For this review, take the finished solid that the model builds, in its own axes (mm). A direction names the side the tool comes from. Round coordinates to 2 decimals unless told otherwise and drop trailing zeros. Order: outer loops, then holes, each group sorted by start corner. A loop starts at its lowest first (then second) coordinate and runs counter-clockwise, first axis right, second up. Notation, with made-up numbers: M 88.5,27 L 141.5,27 A22 ccw 141.5,33 Z; hole C 68,26 d2. An arc over 180 degrees is marked long. Use a Markdown table: item, result.
from build123d import *

# Parameters (mm, degrees)
SKETCH2_W                 = 5
SKETCH2_H                 = 15
BOSS_EXTRUDE1_DEPTH       = 14
BOSS_EXTRUDE1_2_DEPTH     = 14
BOSS_EXTRUDE3_DEPTH       = 25
SKETCH5_W                 = 3
SKETCH5_H                 = 8.8
BOSS_EXTRUDE4_DEPTH       = 14
SKETCH7_W                 = 3
SKETCH7_H                 = 15
BOSS_EXTRUDE5_DEPTH       = 14
SKETCH15_W                = 0.3
SKETCH15_H                = 14
CUT_EXTRUDE2_DEPTH        = 15
SKETCH16_W                = 0.15
SKETCH16_H                = 14
CUT_EXTRUDE3_DEPTH        = 15
FILLET1_R                 = 7
F_4_0MM_DOWEL_HOLE2_D     = 4
FILLET2_R                 = 7
F_4_0MM_DOWEL_HOLE1_D     = 4
F_4_0MM_DOWEL_HOLE1_DEPTH = 26
F_4_0MM_DOWEL_HOLE1_TIP   = 1.201721238
BOSS_EXTRUDE6_DEPTH       = 1
CUT_EXTRUDE4_DEPTH        = 2.4


with BuildPart() as part:
    # Sketch2 → Boss-Extrude1 (new body)
    with BuildSketch(Plane.XY):
        with Locations((-7.5, -1.5)):
            Rectangle(SKETCH2_W, SKETCH2_H)
    extrude(amount=BOSS_EXTRUDE1_DEPTH)



with BuildPart() as body_2:
    # Sketch2 → Boss-Extrude1 2 (new body)
    with BuildSketch(Plane.XY):
        with Locations((7.5, -1.5)):
            Rectangle(SKETCH2_W, SKETCH2_H)
    extrude(amount=BOSS_EXTRUDE1_2_DEPTH)


with BuildPart() as part_1:
    add(part.part)

    add(body_2.part)  # Boss-Extrude3 merges body 2
    # Sketch4 → Boss-Extrude3 (add)
    with BuildSketch(Plane.XY):
        Polygon((-10, 6), (-20, 6), (-22.901603942, 7.206366686), (-26, 7.206366686), (-26, 9.206366686), (-22.502408858, 9.206366686), (-19.600804916, 8), (-10, 8), (10, 8), (19.600804916, 8), (22.502408858, 9.206366686), (26, 9.206366686), (26, 7.206366686), (22.901603942, 7.206366686), (20, 6), (10, 6), align=None)
    extrude(amount=BOSS_EXTRUDE3_DEPTH)

    # Sketch5 → Boss-Extrude4 (add)
    with BuildSketch(Plane.XY):
        with Locations((-11.5, 12.4)):
            Rectangle(SKETCH5_W, SKETCH5_H)
        with Locations((11.5, 12.4)):
            Rectangle(SKETCH5_W, SKETCH5_H)
    extrude(amount=BOSS_EXTRUDE4_DEPTH)

    # Sketch7 → Boss-Extrude5 (add)
    with BuildSketch(Plane.XY):
        with Locations((-14.5, -1.5)):
            Rectangle(SKETCH7_W, SKETCH7_H)
        with Locations((14.5, -1.5)):
            Rectangle(SKETCH7_W, SKETCH7_H)
    extrude(amount=BOSS_EXTRUDE5_DEPTH)

    # Sketch15 → Cut-Extrude2 (cut)
    with BuildSketch(Plane.XZ.offset(9)):
        with Locations((-9.85, 7)):
            Rectangle(SKETCH15_W, SKETCH15_H)
        with Locations((9.85, 7)):
            Rectangle(SKETCH15_W, SKETCH15_H)
        with Locations((-13.15, 7)):
            Rectangle(SKETCH15_W, SKETCH15_H)
        with Locations((13.15, 7)):
            Rectangle(SKETCH15_W, SKETCH15_H)
    extrude(amount=-CUT_EXTRUDE2_DEPTH, mode=Mode.SUBTRACT)

    # Sketch16 → Cut-Extrude3 (cut)
    with BuildSketch(Plane.XZ.offset(9)):
        with Locations((-5.075, 7)):
            Rectangle(SKETCH16_W, SKETCH16_H)
        with Locations((5.075, 7)):
            Rectangle(SKETCH16_W, SKETCH16_H)
    extrude(amount=-CUT_EXTRUDE3_DEPTH, mode=Mode.SUBTRACT)

    # Fillet1
    fillet1_edges = [part_1.edges().sort_by_distance(p)[0] for p in [
        (7.425, -9, 0),
        (7.425, -9, 14),
        (-7.425, -9, 0),
        (-7.425, -9, 14),
        (-14.65, -9, 0),
        (-14.65, -9, 14),
        (14.65, -9, 14),
        (14.65, -9, 0),
    ]]
    fillet(fillet1_edges, radius=FILLET1_R - 0.0001)  # a hair under: the kernel refuses the full size

    # Ø4.0mm Dowel Hole2 (through all)
    with Locations(Plane(origin=(16, 0, 0), x_dir=(0, 0, -1), z_dir=(1, 0, 0))):
        with Locations((-8, -6)):
            Hole(F_4_0MM_DOWEL_HOLE2_D / 2)

    # Fillet2
    fillet2_edges = [part_1.edges().sort_by_distance(p)[0] for p in [
        (-11.5, 16.8, 0),
        (-11.5, 16.8, 14),
        (11.5, 16.8, 0),
        (11.5, 16.8, 14),
    ]]
    fillet(fillet2_edges, radius=FILLET2_R - 0.0001)  # a hair under: the kernel refuses the full size

    # Ø4.0mm Dowel Hole1
    with Locations(Plane(origin=(13, 0, 0), x_dir=(0, 0, -1), z_dir=(1, 0, 0))):
        with Locations((-8, 13.5)):
            Hole(F_4_0MM_DOWEL_HOLE1_D / 2, depth=F_4_0MM_DOWEL_HOLE1_DEPTH)
            with Locations((0, 0, -(F_4_0MM_DOWEL_HOLE1_DEPTH + F_4_0MM_DOWEL_HOLE1_TIP / 2))):  # 118° drill point
                Cone(0, F_4_0MM_DOWEL_HOLE1_D / 2, F_4_0MM_DOWEL_HOLE1_TIP, mode=Mode.SUBTRACT)

    # Sketch14 → Boss-Extrude6 (add)
    with BuildSketch(Plane.XY):
        Polygon((-22.901603942, 7.206366686), (-26, 7.206366686), (-26, -2), (-16, -2), (-16, 6), (-20, 6), align=None)
        Polygon((20, 6), (16, 6), (16, -2), (26, -2), (26, 7.206366686), (22.901603942, 7.206366686), align=None)
    extrude(amount=BOSS_EXTRUDE6_DEPTH)

    # Sketch18 → Cut-Extrude4 (cut)
    with BuildSketch(Plane(origin=(-5.15, 0, 0), x_dir=(0, 0, -1), z_dir=(1, 0, 0))):
        Polygon((-6.110899152, -3.235107358), (-9.449916842, -2.981544355), (-11.33901769, -5.746436996), (-9.889100848, -8.764892642), (-6.550083158, -9.018455645), (-4.66098231, -6.253563004), align=None)
    cut_extrude4 = extrude(amount=-CUT_EXTRUDE4_DEPTH, mode=Mode.SUBTRACT)

    # Mirror1: Cut-Extrude4 across plane
    add(cut_extrude4.mirror(Plane(origin=(0, 0, 0), x_dir=(0, 0, 1), z_dir=(1, 0, 0))), mode=Mode.SUBTRACT)


solid = part_1.part
Q1. Machinability: for faces 1 (the flat face through (6.33, -6.99, 10.74)), 2 (the cylindrical face through (9, -6, 6)), 3 (the flat face through (-21.43, 6.595, 12.832)), 4 (the flat face through (-5.15, 0, 7)), which of the approach directions +Z, -Z, +X, -X, +Y, -Y give a long, thin tool a straight path to every point of the face, cutting with its end or side? Answer none if there is none.
Determined:
| item | result |
|---|---|
| face 1 | none |
| face 2 | +X, -X |
| face 3 | +Z, -X, -Y |
| face 4 | +Z, -Z, -Y |
Q2. Add section D-D (x = 3). Write out the cut boundary in (y, z), then the cut area to 3 significant figures.
Determined:
| item | result |
|---|---|
| outline | M 6,0 L 8,0 L 8,25 L 6,25 Z |
| area | 50.0 mm^2 |
Q3. Add section C-C (z = 20.5). Write out the cut boundary in (x, y), then the cut area to 3 significant figures.
Determined:
| item | result |
|---|---|
| outline | M -26,7.21 L -22.9,7.21 L -20,6 L 20,6 L 22.9,7.21 L 26,7.21 L 26,9.21 L 22.5,9.21 L 19.6,8 L -19.6,8 L -22.5,9.21 L -26,9.21 Z |
| area | 105 mm^2 |
Q4. Clearance check with flat-ended pins moving along their axes: pin 1 (2 mm diameter, centred on x = -7, z = 11, fed in from -Y); pin 2 (6.5 mm diameter, centred on y = -6, z = 8, fed in from +X); pin 3 (1.5 mm diameter, centred on x = 7, z = 22, fed in from -Y); pin 4 (2.5 mm diameter, centred on y = 13.5, z = 8, fed in from -X). State where each tip first meets the part, or that it passes through.
Determined:
| item | result |
|---|---|
| pin 1 | stops at y = -8.26 |
| pin 2 | stops at x = 16 |
| pin 3 | stops at y = 6 |
| pin 4 | passes through |
Q5. Add section A-A (y = 0). Write out the cut boundary in (x, z).
Determined:
| item | result |
|---|---|
| outline | M -26,0 L -13.3,0 L -13.3,14 L -16,14 L -16,1 L -26,1 Z; M -9.7,0 L -5.15,0 L -5.15,14 L -9.7,14 Z; M 5.15,0 L 9.7,0 L 9.7,14 L 5.15,14 Z; M 13.3,0 L 26,0 L 26,1 L 16,1 L 16,14 L 13.3,14 Z |
Q6. Wall thickness on line 1 along X through (y, z) = (-3, 6.5); line 2 along X through (y, z) = (9, 8.5); line 3 along Y through (x, z) = (6, 22): over which ranges is each line inside the solid? List them lowest first. Write a range as [from, to].
Determined:
| item | result |
|---|---|
| line 1 | x = [-16, -13.3], [-9.7, -5.15], [5.15, 9.7], [13.3, 16] |
| line 2 | x = [-26, -22.01], [-13, -10], [10, 13], [22.01, 26] |
| line 3 | y = [6, 8] |
Q7. Draft analysis for pull direction X (two halves, no side actions). For faces 5 (the flat face through (21.47, 6.61, 12.83)), 6 (the flat face through (24, 7.206, 13)), 7 (the flat face through (10, 11, 7)), state which applies: pulls with the +X half, pulls with the -X half, needs draft (parallel to the pull), parting line crosses it, or undercut.
Determined:
| item | result |
|---|---|
| face 5 | pulls with the +X half |
| face 6 | needs draft |
| face 7 | undercut |
